```python
from build123d import *

# Parameters (mm, degrees)
SKETCH1_W           = 60
SKETCH1_H           = 10
BOSS_EXTRUDE1_DEPTH = 2


with BuildPart() as part:
    # Sketch1 → Boss-Extrude1 (new body)
    with BuildSketch(Plane.XY):
        Polygon((90, 0), (0, 0), (0.258301591, -19.998335275), (-1.418256709, -19.998335275), (-0.837659875, -64.994589645), (0.839480171, -64.994589645), (1.097803264, -84.994589645), (-0.579595357, -84.994589645), (0.001001477, -129.990844015), (1.678981844, -129.990844015), (2.001001477, -154.922384552), (88.001001477, -154.922384552), (88.322698776, -129.990844015), (90.001001477, -129.990844015), (90.581598311, -84.994589645), (88.903295611, -84.994589645), (89.161360128, -64.994589645), (90.839662829, -64.994589645), (91.420259663, -19.998335275), (89.741956963, -19.998335275), align=None)
        Polygon((25.324989117, -25), (64.675338274, -25), (63.321501046, -129.922384552), (26.680182862, -129.922384552), align=None, mode=Mode.SUBTRACT)
        with Locations((45.001001477, -11.176996481)):
            Rectangle(SKETCH1_W, SKETCH1_H, mode=Mode.SUBTRACT)
    extrude(amount=BOSS_EXTRUDE1_DEPTH)


solid = part.part
```
For this review, take the finished solid that the model builds, in its own axes (mm). Round coordinates to 2 decimals unless told otherwise and drop trailing zeros. Write each loop counter-clockwise with the first axis right and the second up, starting at its lowest first coordinate (ties: lowest second). Pieces come first, ordered by that corner, then holes.
1) Take a section at D-D on y = -102. Give the boundary of the cut face in (x, z), then the cut area to 3 significant figures.
Answer below:
outline: (-0.36, 0) - (26.32, 0) - (26.32, 2) - (-0.36, 2) - close; (63.68, 0) - (90.36, 0) - (90.36, 2) - (63.68, 2) - close
area: 107 mm2
2) Take a section at A-A on x = 34.5. Give the boundary of the cut face in (y, z).
Answer below:
outline: (-154.92, 0) - (-129.92, 0) - (-129.92, 2) - (-154.92, 2) - close; (-25, 0) - (-16.18, 0) - (-16.18, 2) - (-25, 2) - close; (-6.18, 0) - (0, 0) - (0, 2) - (-6.18, 2) - close
3) For line 1 along Y through (x, z) = (32, 0.25); line 2 along Y through (x, z) = (19.5, 1.7); line 3 along X through (y, z) = (-62, 0.85), list the stretches that pass through material, from the lowest coordinate up.
Answer below:
line 1: y = -154.92 to -129.92, -25 to -16.18, -6.18 to 0
line 2: y = -154.92 to -16.18, -6.18 to 0
line 3: x = -0.88 to 25.8, 64.2 to 90.88
4) Take a section at B-B on x = 23.5. Give the boundary of the cut face in (y, z), then the cut area to 3 significant figures.
Answer below:
outline: (-154.92, 0) - (-16.18, 0) - (-16.18, 2) - (-154.92, 2) - close; (-6.18, 0) - (0, 0) - (0, 2) - (-6.18, 2) - close
area: 290 mm2
5) Take a section at C-C on z = 1.1. Give the boundary of the cut face in (x, y), then the cut area to 3 significant figures.
Answer below:
outline: (-1.42, -20) - (-0.84, -64.99) - (0.84, -64.99) - (1.1, -84.99) - (-0.58, -84.99) - (0, -129.99) - (1.68, -129.99) - (2, -154.92) - (88, -154.92) - (88.32, -129.99) - (90, -129.99) - (90.58, -84.99) - (88.9, -84.99) - (89.16, -64.99) - (90.84, -64.99) - (91.42, -20) - (89.74, -20) - (90, 0) - (0, 0) - (0.26, -20) - close; hole (15, -16.18) - (75, -16.18) - (75, -6.18) - (15, -6.18) - close; hole (25.32, -25) - (26.68, -129.92) - (63.32, -129.92) - (64.68, -25) - close
area: 9,350 mm2
6) Insertion check: pin 1 Ø0.6 at (y, z) = (-10, 1) entering from -X; pin 2 Ø0.8 at (x, z) = (90, 0.5) entering from -Y; pin 3 Ø0.8 at (x, z) = (90.5, 1) entering from +Y; pin 4 Ø0.8 at (x, z) = (0.5, 1) entering from +Y. Each pin has a flat end and moves straight along its axis. Give the tip position at first contact, or say it passes through.
Answer below:
pin 1: stops at x = 0.13
pin 2: stops at y = -129.99
pin 3: stops at y = -20
pin 4: stops at y = 0
